from build123d import *

# Parameters (mm, degrees)
BOSS_EXTRUDE1_DEPTH = 120
FILLET2_R           = 20
SKETCH2_R           = 6
BOSS_EXTRUDE2_DEPTH = 3.5


with BuildPart() as part:
    # Sketch1 → Boss-Extrude1 (new body)
    with BuildSketch(Plane(origin=(0, 0, 0), x_dir=(0, 0, -1), z_dir=(1, 0, 0))):
        Polygon((-70, 0), (0, 0), (0, 60), (-50, 60), align=None)
    extrude(amount=BOSS_EXTRUDE1_DEPTH)

    # Fillet2
    fillet2_edges = [part.edges().sort_by_distance(p)[0] for p in [
        (60, 60, 50),
    ]]
    fillet(fillet2_edges, radius=FILLET2_R)

    # Sketch2 → Boss-Extrude2 (add)
    with BuildSketch(Plane(origin=(0, 21, 63), x_dir=(1, 0, 0), z_dir=(0, 0.316227766016838, 0.9486832980505138))):
        with Locations(Location((13.570097229, -9.935839792, 0), (0, 0, 90))):
            Circle(SKETCH2_R)
        with Locations(Location((106.519183085, -9.935839792, 0), (0, 0, 90))):
            Circle(SKETCH2_R)
    extrude(amount=BOSS_EXTRUDE2_DEPTH)


solid = part.part
Geometry check sheet. Reference: the model listing, model coordinates, mm. Round coordinates to 2 decimals unless told otherwise and drop trailing zeros. Order: outer loops, then holes, each group sorted by start corner. A loop starts at its lowest first (then second) coordinate and runs counter-clockwise, first axis right, second up. Notation, with made-up numbers: M 79.25,-8.5 L 101.25,-8.5 A16 cw 101.25,21.5 Z; hole C 33,71 d11. An arc over 180 degrees is marked long. Write each question's results on one line, items separated by ' | '. Start each with the question number.
1. Cross-section at A-A on x = 111. Record the boundary of the cut face in (y, z), plus the area to 3 significant figures.
2. Draft check along Y on faces 1 (the face through (101.46, 15.18, 66.76)), 2 (the face through (106.44, 12.6, 69.49)), 3 (the face through (59, 0, 35)). Enter one of: pulls with the +Y half, pulls with the -Y half, needs draft (parallel to the pull), parting line crosses it, or undercut.
3. Material ranges on L1, parallel to Z at x = 34, y = 12; L2, parallel to Y at x = 24, z = 39; L3, parallel to Z at x = 104, y = 57, recorded low to high. Write a range as from..to.
4. Go/stop test with a flat-tipped pin: P1, Ø1.5, axis at x = 43, y = 7.5, coming from the +Z side. Record where the tip stops, or that it passes through.
5. Cross-section at C-C on y = 33.5. Record the boundary of the cut face in (x, z).
6. Cross-section at D-D on x = 97. Record the boundary of the cut face in (y, z).
7. Cross-section at B-B on z = 58.5. Record the boundary of the cut face in (x, y).
Resolved:
1) outline: M 0,0 L 60,0 L 60,35.58 A20 ccw 46.32,54.56 L 15.36,64.88 L 16.47,68.2 L 8.9,70.72 L 7.79,67.4 L 0,70 Z | area: 3,590 mm2
2) face 1: undercut | face 2: pulls with the +Y half | face 3: pulls with the -Y half
3) L1: 0..66 | L2: 0..59.71 | L3: 0..46.12
4) P1: z = 67.75
5) outline: M 0,0 L 120,0 L 120,58.83 L 0,58.83 Z
6) outline: M 0,0 L 60,0 L 60,35.58 A20 ccw 46.32,54.56 L 0,70 Z
7) outline: M 0,0 L 120,0 L 120,34.5 L 0,34.5 Z
